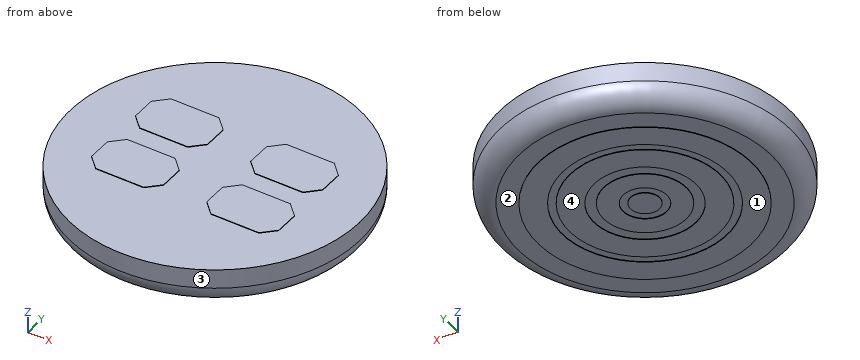
```python
from build123d import *

# Parameters (mm, degrees)
SKETCH_1_R      = 3
EXTRUDE_1_DEPTH = 0.8
SKETCH_2_R      = 2.2
SKETCH_2_R_2    = 1.7
SKETCH_2_R_3    = 1.55
SKETCH_2_R_4    = 1.05
SKETCH_2_R_5    = 0.85
SKETCH_2_R_6    = 0.45
SKETCH_2_R_7    = 0.3
EXTRUDE_2_DEPTH = 0.01
EXTRUDE_3_DEPTH = 0.01
FILLET_2_R      = 0.4


with BuildPart() as part:
    # 草图1 → 凸台-拉伸1 (new body)
    with BuildSketch(Plane.XY):
        Circle(SKETCH_1_R)
    extrude(amount=EXTRUDE_1_DEPTH)

    # 草图2 → 凸台-拉伸2 (add)
    with BuildSketch(Plane(origin=(0, 0, 0), x_dir=(-1, 0, 0), z_dir=(0, 0, -1))):
        with Locations(Location((0, 0, 0), (0, 0, 180))):  # turned: the seam where the file's is
            Circle(SKETCH_2_R)
        Circle(SKETCH_2_R_2, mode=Mode.SUBTRACT)
        with Locations(Location((0, 0, 0), (0, 0, 180))):  # turned: the seam where the file's is
            Circle(SKETCH_2_R_3)
        Circle(SKETCH_2_R_4, mode=Mode.SUBTRACT)
        with Locations(Location((0, 0, 0), (0, 0, 180))):  # turned: the seam where the file's is
            Circle(SKETCH_2_R_5)
        Circle(SKETCH_2_R_6, mode=Mode.SUBTRACT)
        with Locations(Location((0, 0, 0), (0, 0, 180))):  # turned: the seam where the file's is
            Circle(SKETCH_2_R_7)
    extrude(amount=EXTRUDE_2_DEPTH)

    # 草图3 → 凸台-拉伸3 (add)
    with BuildSketch(Plane.XY.offset(0.8)):
        Polygon((-0.45, 0.95), (-0.7, 1.2), (-1.7, 1.2), (-1.95, 0.95), (-1.95, 0.45), (-1.7, 0.2), (-0.7, 0.2), (-0.45, 0.45), align=None)
        Polygon((0.45, 0.95), (0.45, 0.45), (0.7, 0.2), (1.7, 0.2), (1.95, 0.45), (1.95, 0.95), (1.7, 1.2), (0.7, 1.2), align=None)
        Polygon((0.45, -0.95), (0.7, -1.2), (1.7, -1.2), (1.95, -0.95), (1.95, -0.45), (1.7, -0.2), (0.7, -0.2), (0.45, -0.45), align=None)
        Polygon((-0.45, -0.95), (-0.45, -0.45), (-0.7, -0.2), (-1.7, -0.2), (-1.95, -0.45), (-1.95, -0.95), (-1.7, -1.2), (-0.7, -1.2), align=None)
    extrude(amount=EXTRUDE_3_DEPTH)

    # 圆角2
    fillet_2_edges = [part.edges().sort_by_distance(p)[0] for p in [
        (-3, 0, 0),
    ]]
    fillet(fillet_2_edges, radius=FILLET_2_R)


solid = part.part
```
Read the model definition and answer for the solid it produces. Units are mm, in the model's axes. Face numbers are marked on the shaded views. A direction names the side the tool comes from. Give positions to 0.01 mm unless a question says otherwise; leave off trailing zeros. Write each loop counter-clockwise with the first axis right and the second up, starting at its lowest first coordinate (ties: lowest second). Pieces come first, ordered by that corner, then holes. Notation, with made-up numbers: (72.5, -19) - (121.5, -19) arc R22 ccw to (121.5, 15) - close; hole circle Ø4 at (79.25, 66.5). An arc over 180 degrees is marked (long way). Write item = value, one per line. Start each with the question number.
Item 1: Find section C-C (z = 0.65). Give the vertices of the cut face in (x, y), then the cut area to 3 significant figures.
Item 2: The mould has two halves that part along Y. Classify the marked faces 3 and 4: +Y half, -Y half, draft (parallel to the pull), parting line (faces both ways), or undercut.
Item 3: Find section D-D (z = 0.2). Give the vertices of the cut face in (x, y), then the cut area to 3 significant figures.
Item 4: Find the intervals of material crossed by probe 1 along Z at (x, y) = (-0.55, 0.15); probe 2 along X at (y, z) = (-0.1, 0.5); probe 3 along Y at (x, z) = (-1.55, 0.75), in increasing order. Write a range as [from, to].
Item 5: A tool of negligible diameter and unlimited length cuts with its end or side. For the marked faces 1 and 2, from which of +Z, -Z, +X, -X, +Y, -Y can it reach the whole face along a straight path? Write none if from no direction.
Response:
q1.outline = circle Ø6 at (0, 0)
q1.area = 28.3 mm²
q2.face_3 = parting line
q2.face_4 = draft
q3.outline = circle Ø5.89 at (0, 0)
q3.area = 27.3 mm²
q4.probe_1 = [-0.01, 0.8]
q4.probe_2 = [-3, 3]
q4.probe_3 = [-2.57, 2.57]
q5.face_1 = -Z, +X, -X, +Y, -Y
q5.face_2 = -Z
